Input: dimensioned drawing with shaded views. Units: mm. Origin: part minimum x, y, z. A direction names the side the tool comes from. Give positions to 0.01 mm unless a question says otherwise; leave off trailing zeros. Write each loop counter-clockwise with the first axis right and the second up, starting at its lowest first coordinate (ties: lowest second). Pieces come first, ordered by that corner, then holes.
Q1. Section B-B (z = 37.5). Return the cut outline in (x, y).
Q2. Reachability of the marked faces 1, 2 and 3 from +Z, -Z, +X, -X, +Y, -Y: full face, straight path, thin tool, end or side. Return the list, or none.
Q3. Section D-D (x = 45). Return the cut outline in (y, z).
Q4. Section C-C (y = 57). Return the cut outline in (x, z), plus the area to 3 significant figures.
Q5. Section A-A (x = 11.5). Return the cut outline in (y, z), plus the area to 3 significant figures.
Q6. Line query: line 1 (Y direction, x = 33.5, z = 38); line 2 (X direction, y = 83.5, z = 8.5); line 3 (Y direction, x = 85, z = 41.5). Output: solid intervals per line, ascending.
Q7. Pin query (flat end, axial travel): pin 1 Ø13 at (x, z) = (44, 15) entering from +Y; pin 2 Ø9 at (x, y) = (5.5, 65.5) entering from +Z. Return the tip coordinate at first contact, or that it passes through.
Q8. Mould query, pull axis X, two halves, no side actions, for the marked faces 4, 5 and 6. Classes: +X half, -X half, draft (parallel to the pull), parting line (faces both ways), or undercut.
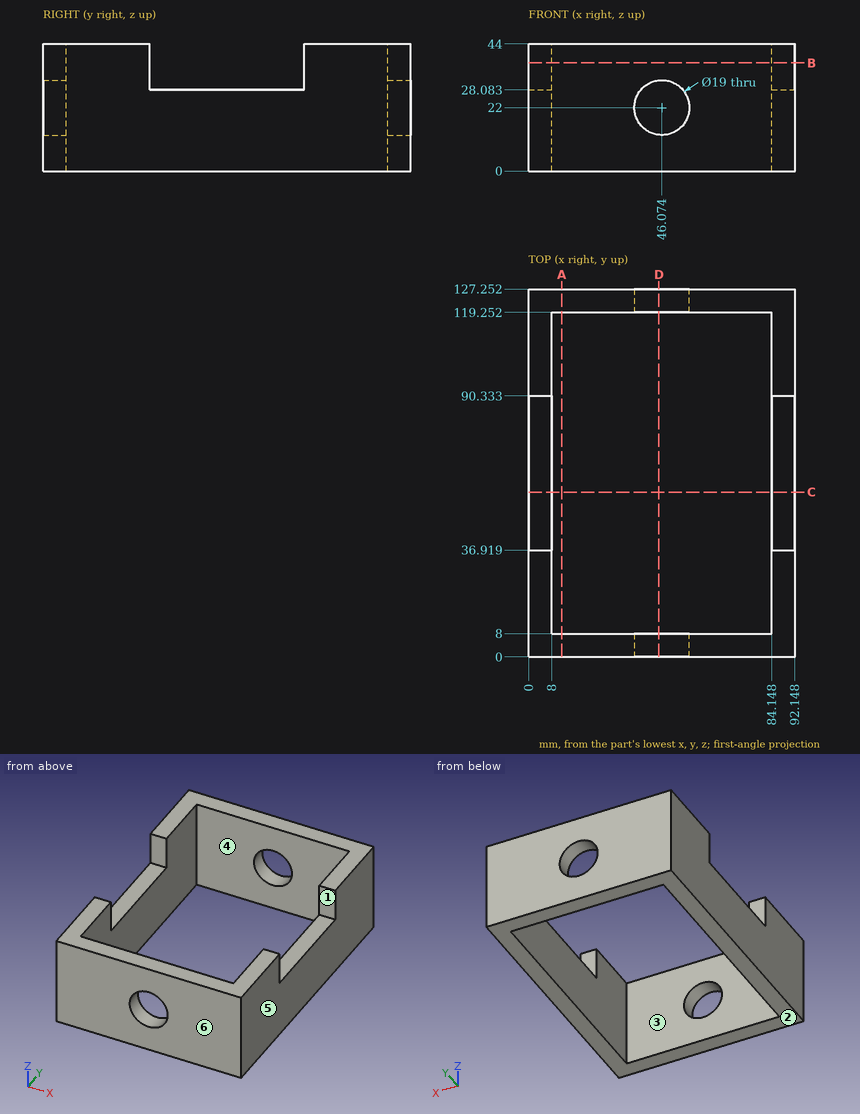
Computed:
1. outline: (0, 0) - (92.15, 0) - (92.15, 36.92) - (84.15, 36.92) - (84.15, 8) - (8, 8) - (8, 36.92) - (0, 36.92) - close; (0, 90.33) - (8, 90.33) - (8, 119.25) - (84.15, 119.25) - (84.15, 90.33) - (92.15, 90.33) - (92.15, 127.25) - (0, 127.25) - close
2. face 1: +Z, +X, -X
2. face 2: -Z, +X, -X, +Y, -Y
2. face 3: +Z, -Z
3. outline: (0, 0) - (8, 0) - (8, 12.56) - (0, 12.56) - close; (0, 31.44) - (8, 31.44) - (8, 44) - (0, 44) - close; (119.25, 0) - (127.25, 0) - (127.25, 12.56) - (119.25, 12.56) - close; (119.25, 31.44) - (127.25, 31.44) - (127.25, 44) - (119.25, 44) - close
4. outline: (0, 0) - (8, 0) - (8, 28.08) - (0, 28.08) - close; (84.15, 0) - (92.15, 0) - (92.15, 28.08) - (84.15, 28.08) - close
4. area: 449 mm2
5. outline: (0, 0) - (8, 0) - (8, 44) - (0, 44) - close; (119.25, 0) - (127.25, 0) - (127.25, 44) - (119.25, 44) - close
5. area: 704 mm2
6. line 1: y = 0 to 8, 119.25 to 127.25
6. line 2: x = 0 to 8, 84.15 to 92.15
6. line 3: y = 0 to 36.92, 90.33 to 127.25
7. pin 1: stops at y = 127.25
7. pin 2: stops at z = 28.08
8. face 4: undercut
8. face 5: +X half
8. face 6: draft
